```python
from build123d import *

# Parameters (mm, degrees)
PAD007_DEPTH         = 2.7
CYLINDER1020_R       = 2.7
CYLINDER1020_DEPTH   = 10
CYLINDER1018_R       = 1.7
CYLINDER1018_DEPTH   = 10
CLONE023_PITCH_ANGLE = 90
CYLINDER1014_R       = 2.7
CYLINDER1014_DEPTH   = 100
CYLINDER1016_R       = 1
CYLINDER1016_DEPTH   = 10
ARRAY_COUNT          = 15
CYLINDER_R           = 13
CYLINDER_DEPTH       = 9.4


with BuildPart() as clone_of_m3nuthousingmaster001:
    # Sketch008 → Pad007 (new body)
    with BuildSketch(Plane(origin=(65, 30, 1.5), x_dir=(0, 0, 1), z_dir=(-1, 0, 0))):
        Polygon((0, 0), (1.674316, 2.9), (21.674316, 2.9), (21.674316, -2.9), (1.674316, -2.9), align=None)
    extrude(amount=PAD007_DEPTH)


with BuildPart() as clone_of_m3nuthousingmaster001_1:
    # Clone010 placement: moved
    add(clone_of_m3nuthousingmaster001.part.moved(Location((-58.3, -30, 0))))


with BuildPart() as cylinder1015:
    # Cylinder1020 → Cylinder1020 (new body)
    with BuildSketch(Plane.XY.offset(10)):
        Circle(CYLINDER1020_R)
    extrude(amount=CYLINDER1020_DEPTH)


with BuildPart() as clone_of_m3bolthead:
    # Cylinder1018 → Cylinder1018 (new body)
    with BuildSketch(Plane.XY):
        Circle(CYLINDER1018_R)
    extrude(amount=CYLINDER1018_DEPTH)

    # Fusion024: union Cylinder1015
    add(cylinder1015.part)


with BuildPart() as clone_of_m3bolthead_1:
    # Clone023 pitch: moved
    add(clone_of_m3bolthead.part.rotate(Axis((0, 0, 0), (0, 1, 0)), CLONE023_PITCH_ANGLE))


with BuildPart() as clone_of_m3bolthead_2:
    # Clone023 placement: moved
    add(clone_of_m3bolthead_1.part.moved(Location((0, 0, 5))))


with BuildPart() as fusion:
    # Cylinder1014 → Cylinder1014 (new body)
    with BuildSketch(Plane.XY):
        Circle(CYLINDER1014_R)
    extrude(amount=CYLINDER1014_DEPTH)

    # Fusion: union Clone of M3NutHousingMaster001, Clone of M3BoltHead
    add(clone_of_m3nuthousingmaster001_1.part)
    add(clone_of_m3bolthead_2.part)


with BuildPart() as array:
    # Cylinder1016 → Cylinder1016 (new body)
    with BuildSketch(Plane(origin=(0, 13.5, 0), x_dir=(1, 0, 0), z_dir=(0, 0, 1))):
        Circle(CYLINDER1016_R)
    extrude(amount=CYLINDER1016_DEPTH)

    # Array: Array ×15 about axis
    array_axis = Axis((0, 0, 0), (0, 0, 1))


with BuildPart() as array_1:
    add(array.part)
    for i in range(1, ARRAY_COUNT):
        add(array.part.rotate(array_axis, i * 360 / ARRAY_COUNT))


with BuildPart() as wheel:
    # Cylinder → Cylinder (new body)
    with BuildSketch(Plane.XY):
        Circle(CYLINDER_R)
    extrude(amount=CYLINDER_DEPTH)

    # Cut013: cut Array
    add(array_1.part, mode=Mode.SUBTRACT)

    # Cut019: cut Fusion
    add(fusion.part, mode=Mode.SUBTRACT)


solid = wheel.part
```
Source: CAD feature listing. Evaluate the final solid. Frame: model axes, mm. A direction names the side the tool comes from. Round coordinates to 2 decimals unless told otherwise and drop trailing zeros. Loops run counter-clockwise (first coordinate to the right, second up) from the corner with the lowest first, then second, coordinate; pieces in that order, holes last. Notation, with made-up numbers: M 16,44 L 53,44 A31 cw 53,78 Z; hole C 11,0.25 d1. An arc over 180 degrees is marked long. Use a Markdown table: item, result. Add a question column.
1. Cut plane A-A, the plane x = 0. Output: boundary loops of the cut face in (y, z).
2. Cut plane B-B, the plane x = 11.25. Output: boundary loops of the cut face in (y, z).
3. Contact query for flat-ended pins moving along their axis: pin 1 (3 mm diameter, centred on x = 5.5, z = 7.5, fed in from +Y); pin 2 (3 mm diameter, centred on y = 8.5, z = 7, fed in from -X); pin 3 (10 mm diameter, centred on x = -9.5, y = -1.5, fed in from -Z); pin 4 (1 mm diameter, centred on y = -3.5, z = 4.5, fed in from +X). Output: stop coordinate, or through.
4. Cut plane C-C, the plane z = 8.25. State how many separate pieces and enclosed holes the cut face has, and give its area (3 significant figures).
5. Set-up query: faces 1 (the cylindrical face through (11.479, 2.677, 5.351)), 2 (the flat face through (6.7, 0, 7)), 3 (the cylindrical face through (12.356, -4.042, 4.634)). Return all of +Z, -Z, +X, -X, +Y, -Y with unobstructed straight access to the full face (end or side cutting, diameter ignored); none if empty.
6. Ray query, line 1 along Z through (x, y) = (8.9, 0); line 2 along Z through (x, y) = (12.3, 0); line 3 along Y through (x, z) = (3.1, 5). Return the intervals inside material, ascending. Write a range as [from, to].
7. Pull-direction query (X, two-part tool) for faces 4 (the cylindrical face through (-2.59, -12.23, 4.63)), 5 (the flat face through (10, 0, 3)), 6 (the cylindrical face through (-2.7, 0.1, 4.6)), 7 (the flat face through (0, -3, 9.4)); classes: +X half, -X half, draft (parallel to the pull), parting line (faces both ways), or undercut.
8. Cut plane D-D, the plane y = 9.75. Output: boundary loops of the cut face in (x, z), and give its area (3 significant figures).
Solution:
| question | item | result |
|---|---|---|
| 1 | outline | M -13,0 L -2.7,0 L -2.7,9.4 L -13,9.4 Z; M 2.7,0 L 12.5,0 L 12.5,9.4 L 2.7,9.4 Z |
| 2 | outline | M -5.85,0 L 6.51,0 L 6.51,9.4 L -5.85,9.4 Z; hole C 0,5 d5.4 |
| 3 | pin 1 | stops at y = 12.37 |
| 3 | pin 2 | stops at x = -10.95 |
| 3 | pin 3 | stops at z = 0 |
| 3 | pin 4 | stops at x = 12.65 |
| 4 | separate pieces | 1 |
| 4 | enclosed holes | 2 |
| 4 | area | 483 mm2 |
| 5 | face 1 | +X |
| 5 | face 2 | +Z |
| 5 | face 3 | +Z, -Z, +X, -Y |
| 6 | line 1 | z = [0, 3.3], [6.7, 9.4] |
| 6 | line 2 | z = [0, 2.3], [7.7, 9.4] |
| 6 | line 3 | y = [-12.25, -1.7], [1.7, 12.62] |
| 7 | face 4 | undercut |
| 7 | face 5 | +X half |
| 7 | face 6 | undercut |
| 7 | face 7 | draft |
| 8 | outline | M -8.6,0 L 8.6,0 L 8.6,9.4 L -8.6,9.4 Z |
| 8 | area | 162 mm2 |
